from build123d import *

# Parameters (mm, degrees)
F1_DEPTH       = 3.175
F2_D           = 2.54
F2_CSINK_D     = 9.525
F2_CSINK_ANGLE = 90
F3_D           = 7.62
F3_CSINK_D     = 9.525
F3_CSINK_ANGLE = 90


with BuildPart() as f1:
    # F0 (on Front) → F1 (new body)
    with BuildSketch(Plane.XZ):
        with BuildLine():
            Line((6.35, 0), (6.35, 88.9))
            Line((6.35, 88.9), (-6.35, 88.9))
            Line((-6.35, 88.9), (-6.35, 0))
            ThreePointArc((-6.35, 0), (0, -6.35), (6.35, 0))
        make_face()
    extrude(amount=F1_DEPTH)

    # F2 (through all)
    with Locations(Plane(origin=(0, 0, 0), x_dir=(1, 0, 0), z_dir=(0, 1, 0))):
        with Locations((0, -82.55), (0, -61.9125), (0, -30.1625)):
            CounterSinkHole(F2_D / 2, F2_CSINK_D / 2, counter_sink_angle=F2_CSINK_ANGLE)

    # F3 (through all)
    with Locations(Plane(origin=(0, 0, 0), x_dir=(1, 0, 0), z_dir=(0, 1, 0))):
        with Locations((0, 0)):
            CounterSinkHole(F3_D / 2, F3_CSINK_D / 2, counter_sink_angle=F3_CSINK_ANGLE)


solid = f1.part
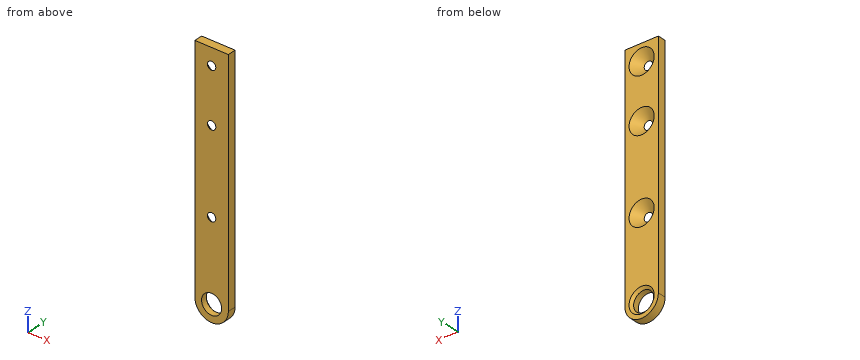
Read the model definition and answer for the solid it produces. Units are mm, in the model's axes. Round coordinates to 2 decimals unless told otherwise and drop trailing zeros.
1) A flat-ended cylindrical pin translates along its axis: pin 1 (4 mm diameter, centred on x = 0, z = 27.5, fed in from +Y). Find the tip coordinate at first contact, or state that the pin passes through.
2) Straight lines are drawn through the part: L1, parallel to Z at x = 0.5, y = -2.45; L2, parallel to Z at x = -2, y = -0.65; L3, parallel to X at y = -0.3, z = 31. For each, find the intervals that lie inside material, in ascending order.
3) The part is cut by section A-A on x = 0. Give the number of separate pieces and of enclosed holes in the cut face, plus the area to 3 significant figures.
Resolved:
1. pin 1: stops at y = -0.1
2. L1: z = -6.33 to -3.78, 3.78 to 27.9, 32.42 to 59.65, 64.17 to 80.29, 84.81 to 88.9
2. L2: z = -6.03 to -3.59, 3.59 to 26.57, 33.76 to 58.32, 65.51 to 78.96, 86.14 to 88.9
2. L3: x = -6.35 to -4.38, 4.38 to 6.35
3. separate pieces: 5
3. enclosed holes: 0
3. area: 217 mm2
